from build123d import *


with BuildPart() as part:
    # Sweep1: sweep along a path in Sketch2
    with BuildLine(Plane(origin=(2.5, 0, 0), x_dir=(0, 0, -1), z_dir=(1, 0, 0))) as sweep1_path:
        Line((150, 92), (-150, 92))
        ThreePointArc((-150, 92), (-165.556349186, 85.556349186), (-172, 70))
        Line((-172, 70), (-172, -70))
        ThreePointArc((-172, -70), (-165.556349186, -85.556349186), (-150, -92))
        Line((-150, -92), (150, -92))
        ThreePointArc((150, -92), (165.556349186, -85.556349186), (172, -70))
        Line((172, -70), (172, 70))
        ThreePointArc((172, 70), (165.556349186, 85.556349186), (150, 92))
    # Sketch1 → Sweep1 (sweep)
    with BuildSketch(Plane.XY):
        with BuildLine():
            Line((5, 81), (5, 89.5))
            ThreePointArc((5, 89.5), (4.267766953, 91.267766953), (2.5, 92))
            ThreePointArc((2.5, 92), (0.732233047, 91.267766953), (0, 89.5))
            Line((0, 89.5), (0, 82.5))
            ThreePointArc((0, 82.5), (-0.732233047, 80.732233047), (-2.5, 80))
            ThreePointArc((-2.5, 80), (-4.267766953, 79.267766953), (-5, 77.5))
            Line((-5, 77.5), (-5, 71))
            Line((-5, 71), (-6, 71))
            Line((-6, 71), (-6, 81))
            Line((-6, 81), (-3, 81))
            Line((-3, 81), (-3, 96))
            Line((-3, 96), (8, 96))
            Line((8, 96), (8, 81))
            Line((8, 81), (5, 81))
        make_face()
    sweep(path=sweep1_path.line)


solid = part.part
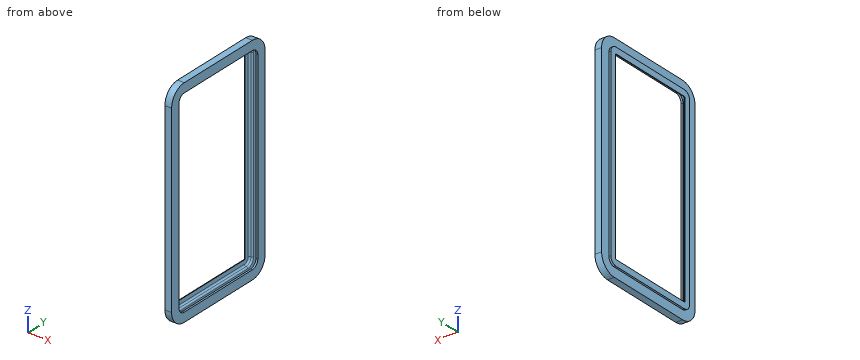
Can you work these out from the model? Positions are in its coordinate system, mm. Coordinates: 2 decimals unless noted, no trailing zeros. Order: outer loops, then holes, each group sorted by start corner. A loop starts at its lowest first (then second) coordinate and runs counter-clockwise, first axis right, second up. Notation, with made-up numbers: (30.5, 36.5) - (46.5, 36.5) arc R16 cw to (46.5, 62.5) - close; hole circle Ø2 at (39.5, 31). An arc over 180 degrees is marked (long way). Answer as a JSON object with one key per item and string values. Group by question number.
Q1. Imagine slicing it at B-B (z = 11). Please give me the cut outline in (x, y).
Q2. Imagine slicing it at A-A (y = 4). Please give me the cut outline in (x, z).
Q3. I need wall thicknesses on line 1 (Y direction, x = 6, z = -93.5); line 2 (Z direction, x = 2, y = -43); line 3 (Y direction, x = -2.5, z = -143). Which ranges of each line are inside material? Lowest first, please. Write a range as from..to.
Q4. Will these pins go through, and if not, where does the flat tip stop? P1, Ø0.8, axis at x = -5.5, z = -2.5, coming from the -Y side; P2, Ø1.1, axis at x = -5.5, y = 17, coming from the +Z side; P3, Ø0.9, axis at x = -4.5, z = 72.5, coming from the +Y side.
Determined:
{
 "1": {"outline": "(-6, -81) - (-3, -81) - (-3, -96) - (8, -96) - (8, -81) - (5, -81) - (5, -89.5) arc R2.5 cw to (0, -89.5) - (0, -82.5) arc R2.5 ccw to (-2.5, -80) arc R2.5 cw to (-5, -77.5) - (-5, -71) - (-6, -71) - close; (-6, 71) - (-5, 71) - (-5, 77.5) arc R2.5 cw to (-2.5, 80) arc R2.5 ccw to (0, 82.5) - (0, 89.5) arc R2.5 cw to (5, 89.5) - (5, 81) - (8, 81) - (8, 96) - (-3, 96) - (-3, 81) - (-6, 81) - close"},
 "2": {"outline": "(-6, -161) - (-3, -161) - (-3, -176) - (8, -176) - (8, -161) - (5, -161) - (5, -169.5) arc R2.5 cw to (0, -169.5) - (0, -162.5) arc R2.5 ccw to (-2.5, -160) arc R2.5 cw to (-5, -157.5) - (-5, -151) - (-6, -151) - close; (-6, 151) - (-5, 151) - (-5, 157.5) arc R2.5 cw to (-2.5, 160) arc R2.5 ccw to (0, 162.5) - (0, 169.5) arc R2.5 cw to (5, 169.5) - (5, 161) - (8, 161) - (8, 176) - (-3, 176) - (-3, 161) - (-6, 161) - close"},
 "3": {"line 1": "y = -96..-81, 81..96", "line 2": "z = -176..-171.95, 171.95..176", "line 3": "y = -96..-80, 80..96"},
 "4": {"P1": "stops at y = -81", "P2": "stops at z = 161", "P3": "stops at y = 81"}
}
